Source: CAD feature listing. Evaluate the final solid. Frame: model axes, mm. Face numbers are marked on the shaded views. A direction names the side the tool comes from. Round coordinates to 2 decimals unless told otherwise and drop trailing zeros. Loops run counter-clockwise (first coordinate to the right, second up) from the corner with the lowest first, then second, coordinate; pieces in that order, holes last. Notation, with made-up numbers: (-19.5, -12.75) -> (-11.5, -12.75) arc R20 cw to (-11.5, 4.25) -> close; hole circle Ø7 at (-15, 75). An arc over 180 degrees is marked (long way). Return JSON: item names as keys, results as strings. Group by question number.
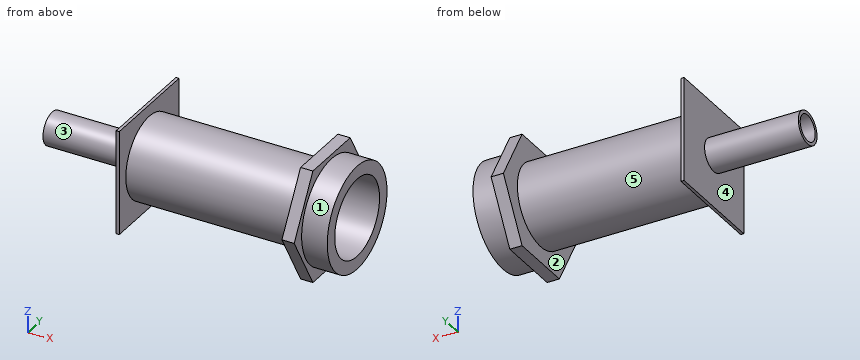
```python
from build123d import *

# Parameters (mm, degrees)
F0_W      = 101.6
F0_H      = 3.175
F3_W      = 101.6
F3_H      = 101.6
F3_R      = 14.2875
F4_DEPTH  = 3
F5_R      = 39.6875
F5_R_2    = 38.1
F6_DEPTH  = 203.2
F7_R      = 50.8
F7_R_2    = 39.6875
F8_DEPTH  = 25
F9_R      = 39.668
F10_DEPTH = 12


with BuildPart() as f1:
    # F0 (on Front) → F1 (revolve)
    with BuildSketch(Plane.XZ):
        with Locations((50.8, 14.2875)):
            Rectangle(F0_W, F0_H)
    revolve(axis=Axis((107.303783, 0, 0), (1, 0, 0)))

    # F3 (on offset) → F4 (join)
    with BuildSketch(Plane.YZ.offset(91.6)):
        Rectangle(F3_W, F3_H)
        Circle(F3_R, mode=Mode.SUBTRACT)
    extrude(amount=F4_DEPTH)

    # F5 (on face) → F6 (join)
    with BuildSketch(Plane.YZ.offset(94.6)):
        Circle(F5_R)
        Circle(F5_R_2, mode=Mode.SUBTRACT)
    extrude(amount=F6_DEPTH)

    # F7 (on face) → F8 (join)
    with BuildSketch(Plane.YZ.offset(297.8)):
        Circle(F7_R)
        Circle(F7_R_2, mode=Mode.SUBTRACT)
    extrude(amount=-F8_DEPTH)

    # F9 (on face) → F10 (join)
    with BuildSketch(Plane(origin=(272.8, 0, 0), x_dir=(0, -1, 0), z_dir=(-1, 0, 0))):
        Polygon((63.50853, 0), (31.754265, 55), (-31.754265, 55), (-63.50853, 0), (-31.754265, -55), (31.754265, -55), align=None)
        Circle(F9_R, mode=Mode.SUBTRACT)
    extrude(amount=F10_DEPTH)


solid = f1.part
```
(1) Cut plane D-D (y = 45). Return loops of the section in (x, z), and give its area (3 significant figures).
(2) Set-up query: the marked faces 1 and 2. Return all of +Z, -Z, +X, -X, +Y, -Y with unobstructed straight access to the full face (end or side cutting, diameter ignored); none if empty.
(3) Pin query (flat end, axial travel): pin 1 (2 mm diameter, centred on x = 135, z = -31, fed in from -Y); pin 2 (2.5 mm diameter, centred on x = 93, y = -3.5, fed in from +Z); pin 3 (6 mm diameter, centred on x = 137.5, z = -18.5, fed in from -Y); pin 4 (12 mm diameter, centred on y = -3.5, z = -2.5, fed in from -X). Return the tip coordinate at first contact, or that it passes through.
(4) Cut plane B-B (x = 30). Return loops of the section in (y, z) (3 decimals), and give its area (3 significant figures).
(5) Mould query, pull axis X, two halves, no side actions, for the marked faces 3, 4 and 5. Classes: released by +X, released by -X, zero draft, split by the parting line, or undercut.
(6) Ray query, line 1 (X direction, y = 8, z = 47); line 2 (Z direction, x = 220, y = 0); line 3 (X direction, y = 47, z = 20.5). Return the intervals inside material, ascending.
(7) Cut plane C-C (z = 22). Return loops of the section in (x, y).
Answers follow:
{
 "1": {"outline": "(91.6, -50.8) -> (94.6, -50.8) -> (94.6, 50.8) -> (91.6, 50.8) -> close; (260.8, -32.06) -> (272.8, -32.06) -> (272.8, -23.57) -> (297.8, -23.57) -> (297.8, 23.57) -> (272.8, 23.57) -> (272.8, 32.06) -> (260.8, 32.06) -> close", "area": "2,250 mm^2"},
 "2": {"face 1": "+X", "face 2": "none"},
 "3": {"pin 1": "y = -25.98", "pin 2": "z = 50.8", "pin 3": "y = -36.54", "pin 4": "through"},
 "4": {"outline": "circle Ø31.75 at (0, 0); hole circle Ø25.4 at (0, 0)", "area": "285 mm^2"},
 "5": {"face 3": "zero draft", "face 4": "released by -X", "face 5": "undercut"},
 "6": {"line 1": "91.6 to 94.6, 260.8 to 297.8", "line 2": "-39.69 to -38.1, 38.1 to 39.69", "line 3": "91.6 to 94.6, 260.8 to 272.8"},
 "7": {"outline": "(91.6, -50.8) -> (94.6, -50.8) -> (94.6, -33.03) -> (260.8, -33.03) -> (260.8, -50.81) -> (272.8, -50.81) -> (272.8, -45.79) -> (297.8, -45.79) -> (297.8, -31.11) -> (94.6, -31.11) -> (94.6, 31.11) -> (297.8, 31.11) -> (297.8, 45.79) -> (272.8, 45.79) -> (272.8, 50.81) -> (260.8, 50.81) -> (260.8, 33.03) -> (94.6, 33.03) -> (94.6, 50.8) -> (91.6, 50.8) -> close"}
}
